Can you work these out from the drawing? Everything is in mm from the part's minimum corner. A direction names the side the tool comes from. Coordinates: 2 decimals unless noted, no trailing zeros. Write each loop counter-clockwise with the first axis right and the second up, starting at its lowest first coordinate (ties: lowest second). Pieces come first, ordered by that corner, then holes. Notation, with made-up numbers: M 51.5,3.5 L 88.5,3.5 A26 ccw 88.5,30.5 Z; hole C 78,39.25 d1. An arc over 180 degrees is marked long. Write item = value, one per line.
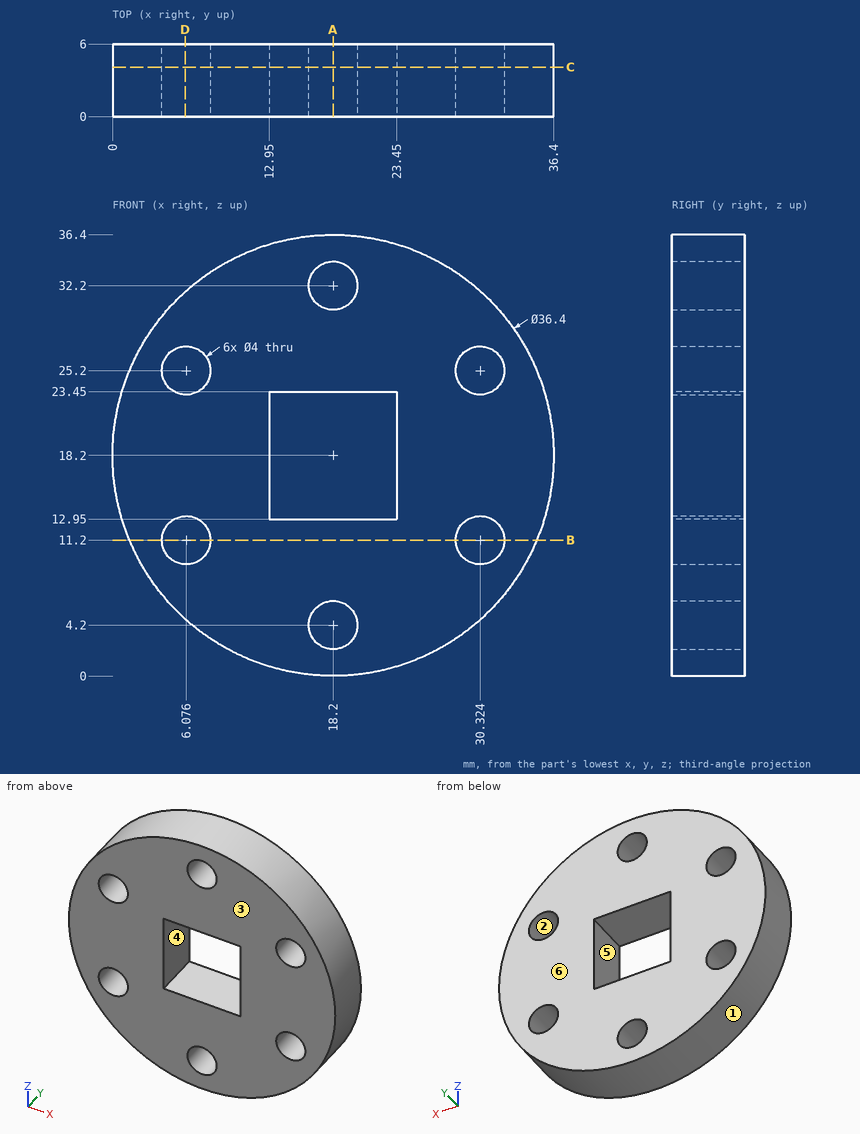
Item 1: Imagine slicing it at A-A (x = 18.2). Write out the boundary of the cut face in (y, z).
Numbers:
outline = M 0,0 L 6,0 L 6,2.2 L 0,2.2 Z; M 0,6.2 L 6,6.2 L 6,12.95 L 0,12.95 Z; M 0,23.45 L 6,23.45 L 6,30.2 L 0,30.2 Z; M 0,34.2 L 6,34.2 L 6,36.4 L 0,36.4 Z
Item 2: If I drill on line 1 along Z through (x, y) = (18.2, 3.1); line 2 along X through (y, z) = (2.5, 11) (1 decimal); line 3 along X through (y, z) = (3.55, 11.5), over which ranges is the centre line in solid material (lowest first)?
Numbers:
line_1 = 0 to 2.2, 6.2 to 12.95, 23.45 to 30.2, 34.2 to 36.4
line_2 = 1.5 to 4.1, 8.1 to 28.3, 32.3 to 34.9
line_3 = 1.28 to 4.1, 8.05 to 28.35, 32.3 to 35.12
Item 3: Imagine slicing it at B-B (z = 11.2). Write out the boundary of the cut face in (x, y) (1 decimal), and give its area (3 significant figures).
Numbers:
outline = M 1.4,0 L 4.1,0 L 4.1,6 L 1.4,6 Z; M 8.1,0 L 28.3,0 L 28.3,6 L 8.1,6 Z; M 32.3,0 L 35,0 L 35,6 L 32.3,6 Z
area = 154 mm²
Item 4: Imagine slicing it at C-C (y = 4.1). State how many separate pieces and enclosed holes the cut face has, and give its area (3 significant figures).
Numbers:
separate_pieces = 1
enclosed_holes = 7
area = 855 mm²
Item 5: For the marked faces 5 and 6, which set-ups out of +Z, -Z, +X, -X, +Y, -Y let a thin tool reach every point of the face, with its end or its side?
Numbers:
face_5 = +Y, -Y
face_6 = +Z, -Z, +X, -X, +Y
Item 6: Imagine slicing it at D-D (x = 6). Write out the boundary of the cut face in (y, z) (1 decimal), and give its area (3 significant figures).
Numbers:
outline = M 0,4.7 L 6,4.7 L 6,9.2 L 0,9.2 Z; M 0,13.2 L 6,13.2 L 6,23.2 L 0,23.2 Z; M 0,27.2 L 6,27.2 L 6,31.7 L 0,31.7 Z
area = 114 mm²
Item 7: I'm going to push flat-ended pins straight in: P1, Ø1.5, axis at x = 26, y = 4, coming from the -Z side; P2, Ø3, axis at y = 3.5, z = 16.5, coming from the -X side. Where does each tip first touch, or does it pass through?
Numbers:
P1 = 1.42
P2 = 0
Item 8: If we mould it in two halves opening along X, with no side actions, what happens to the marked faces 1, 2, 3 and 4? For each: pulls with the +X half, pulls with the -X half, needs draft (parallel to the pull), parting line crosses it, or undercut.
Numbers:
face_1 = parting line crosses it
face_2 = undercut
face_3 = needs draft
face_4 = undercut
